from build123d import *

# Parameters (mm, degrees)
SKETCH1_W           = 12.7
SKETCH1_H           = 9.525
BOSS_EXTRUDE1_DEPTH = 2.54
FILLET1_R           = 0.635
SHELL1_START        = 0.635
SHELL1_OUTLINE_W    = 1.905
SHELL1_OUTLINE_H    = 8.255
SHELL1_DEPTH        = 11.43
SKETCH2_R           = 2.54
BOSS_EXTRUDE2_DEPTH = 1.905
BOSS_EXTRUDE3_DEPTH = 0.00254


# Read off the part's stored shape, not the designer's step: Shell1
with BuildPart() as part:
    # Sketch1 → Boss-Extrude1 (new body)
    with BuildSketch(Plane(origin=(0, 0, 0), x_dir=(1, 0, 0), z_dir=(0, 1, 0))):
        with Locations((6.35, 4.7625)):
            Rectangle(SKETCH1_W, SKETCH1_H)
    extrude(amount=BOSS_EXTRUDE1_DEPTH)

    # Fillet1
    fillet1_edges = [part.edges().sort_by_distance(p)[0] for p in [
        (0, 1.27, -9.525),
        (12.7, 1.27, -9.525),
        (12.7, 1.27, 0),
        (0, 1.27, 0),
    ]]
    fillet(fillet1_edges, radius=FILLET1_R)

    # Shell1 outline → Shell1 (cut)
    with BuildSketch(Plane.YZ.offset(SHELL1_START)):
        with Locations((0.9525, -4.7625)):
            Rectangle(SHELL1_OUTLINE_W, SHELL1_OUTLINE_H)
    extrude(amount=SHELL1_DEPTH, mode=Mode.SUBTRACT)

    # Sketch2 → Boss-Extrude2 (add)
    with BuildSketch(Plane(origin=(0, 1.905, 0), x_dir=(-1, 0, 0), z_dir=(0, -1, 0))):
        with Locations(Location((-6.35, 4.7625, 0), (0, 0, 270))):
            Circle(SKETCH2_R)
    extrude(amount=BOSS_EXTRUDE2_DEPTH)

    # Sketch3 → Boss-Extrude3 (add)
    # profile 1 of 3: a face of its own
    with BuildSketch(Plane(origin=(0, 2.54, 0), x_dir=(1, 0, 0), z_dir=(0, 1, 0))):
        Polygon((3.414346154, 6.477), (4.961141026, 6.477), (4.961141026, 5.907128205), (3.984217949, 5.907128205), (3.984217949, 5.296551282), (4.961141026, 5.296551282), (4.961141026, 4.726679487), (3.984217949, 4.726679487), (3.984217949, 3.302), (3.414346154, 3.302), align=None)
    # profile 2 of 3: a face of its own
    with BuildSketch(Plane(origin=(0, 2.54, 0), x_dir=(1, 0, 0), z_dir=(0, 1, 0))):
        Polygon((5.871282252, 6.477), (6.752166667, 6.477), (6.752166667, 3.302), (6.182294872, 3.302), (6.182294872, 5.947833333), (5.531012821, 5.947833333), align=None)
    # profile 3 of 3: a face of its own
    with BuildSketch(Plane(origin=(0, 2.54, 0), x_dir=(1, 0, 0), z_dir=(0, 1, 0))):
        with BuildLine():
            add(Edge.make_bspline(
                [(8.798235377, 6.558410256), (8.825819537, 6.558000762), (8.880057365, 6.557195586), (8.959939478, 6.548474876), (9.036888038, 6.535300314), (9.111204078, 6.516926396), (9.182352664, 6.492609168), (9.25085163, 6.463501864), (9.31588564, 6.428077745), (9.378284086, 6.388064384), (9.438022931, 6.342763586), (9.493666394, 6.291118337), (9.546230643, 6.234316997), (9.594577855, 6.171500832), (9.639778695, 6.10324122), (9.68168464, 6.029527338), (9.719974889, 5.949998406), (9.755078585, 5.864510908), (9.786468421, 5.771783423), (9.812908041, 5.670752326), (9.83558444, 5.561394546), (9.85472492, 5.443437874), (9.869192029, 5.316725518), (9.878943152, 5.181341659), (9.885634834, 5.037547297), (9.886180963, 4.938905546), (9.886461538, 4.888227965)],
                knots=[0, 0, 0, 0, 0.879237366, 1.728815576, 2.559023295, 3.367336655, 4.166867292, 4.954216142, 5.737608147, 6.525189134, 7.316157332, 8.124696809, 8.942788509, 9.781158001, 10.649253743, 11.551476218, 12.482711956, 13.461909668, 14.496590415, 15.601789533, 16.789733467, 18.056700938, 19.410929216, 20.8549011, 22.384193279, 24, 24, 24, 24], degree=3))
            add(Edge.make_bspline(
                [(9.886461538, 4.888227965), (9.886158312, 4.83691635), (9.885569149, 4.737218804), (9.879221327, 4.592109226), (9.86829008, 4.455742398), (9.854201098, 4.32813243), (9.834903048, 4.20934671), (9.812302348, 4.099077662), (9.785445387, 3.997365257), (9.75302158, 3.904438674), (9.718130367, 3.818801041), (9.679735377, 3.739427172), (9.63850583, 3.666102077), (9.595387407, 3.59771955), (9.548016197, 3.53629547), (9.498697891, 3.4797411), (9.445285081, 3.430210667), (9.390026654, 3.385151595), (9.330898269, 3.346211514), (9.268509703, 3.312155161), (9.201748675, 3.284531414), (9.131832125, 3.260505754), (9.057568312, 3.243257923), (8.980137277, 3.229572336), (8.89866484, 3.222008841), (8.843195123, 3.221070539), (8.814771835, 3.220589744)],
                knots=[0, 0, 0, 0, 1.643780988, 3.193836972, 4.651895693, 6.025988579, 7.305620092, 8.505800249, 9.631074763, 10.672816429, 11.65661981, 12.592235626, 13.49536222, 14.350718032, 15.179365177, 15.97804903, 16.751647189, 17.51006938, 18.259804725, 19.016521909, 19.783502495, 20.571750527, 21.382245291, 22.22305063, 23.089471752, 24, 24, 24, 24], degree=3))
            add(Edge.make_bspline(
                [(8.814771835, 3.220589744), (8.786349314, 3.221079814), (8.730670013, 3.222039854), (8.648977266, 3.229516098), (8.571135886, 3.243313364), (8.496284527, 3.26063817), (8.424944142, 3.284478255), (8.356772657, 3.312928485), (8.292294252, 3.346772343), (8.231330396, 3.38580315), (8.174089237, 3.430560743), (8.119681247, 3.480566389), (8.068226781, 3.535693336), (8.020508587, 3.596559051), (7.975745182, 3.662351105), (7.934403375, 3.733820811), (7.896508012, 3.810864109), (7.86087372, 3.893588392), (7.82991203, 3.983774617), (7.802357564, 4.082228137), (7.779785671, 4.189769642), (7.761631843, 4.306364584), (7.747137838, 4.431765951), (7.736355964, 4.566034271), (7.729972884, 4.709232083), (7.729389899, 4.807659072), (7.729089744, 4.858335136)],
                knots=[0, 0, 0, 0, 0.917216111, 1.796812873, 2.643793957, 3.46689424, 4.273913431, 5.068098542, 5.848489301, 6.620921603, 7.401012384, 8.190319798, 9.003608147, 9.831726257, 10.68377682, 11.569763213, 12.493818149, 13.453288342, 14.474581811, 15.568529029, 16.750744269, 18.018426408, 19.375425659, 20.823733699, 22.36466933, 24, 24, 24, 24], degree=3))
            add(Edge.make_bspline(
                [(7.729089744, 4.858335136), (7.729633447, 4.928745538), (7.730682529, 5.064603314), (7.74397727, 5.2608783), (7.763490579, 5.442300526), (7.792151006, 5.608566515), (7.827589229, 5.760292069), (7.872969718, 5.896477699), (7.924632103, 6.019007839), (7.968655093, 6.091595432), (7.989856971, 6.126554287)],
                knots=[0, 0, 0, 0, 1.288568992, 2.486310467, 3.599230591, 4.627010532, 5.572937695, 6.447898582, 7.252493626, 8, 8, 8, 8], degree=3))
            add(Edge.make_bspline(
                [(7.989856971, 6.126554287), (8.014509505, 6.160897855), (8.062710067, 6.228046298), (8.146990098, 6.316199652), (8.237538017, 6.391592717), (8.336213628, 6.452519281), (8.441456335, 6.500565973), (8.5541697, 6.534500812), (8.673937491, 6.554272829), (8.756184031, 6.557010519), (8.798235377, 6.558410256)],
                knots=[0, 0, 0, 0, 1.058512271, 2.069600068, 3.047294572, 4.004278952, 4.967380941, 5.939006123, 6.946246673, 8, 8, 8, 8], degree=3))
        make_face()
        with BuildLine():
            add(Edge.make_bspline(
                [(8.812227764, 5.988538462), (8.787291455, 5.98735653), (8.738403051, 5.985039317), (8.667463648, 5.965369447), (8.600572221, 5.934988272), (8.549689698, 5.898429277), (8.511604636, 5.863383097), (8.48499433, 5.831667444), (8.459332884, 5.796275061), (8.436667403, 5.755608871), (8.415265272, 5.711130059), (8.394348939, 5.662636719), (8.377203038, 5.608937747), (8.360357645, 5.550947646), (8.345599509, 5.487063142), (8.333235426, 5.41676205), (8.322189206, 5.339587196), (8.314484335, 5.25548803), (8.307301083, 5.164552541), (8.302151788, 5.06657816), (8.299998997, 4.961591317), (8.29931469, 4.889288437), (8.298961538, 4.85197496)],
                knots=[0, 0, 0, 0, 1.076674018, 2.110852608, 3.161083442, 4.239746716, 4.804137807, 5.395870207, 6.026861976, 6.692161227, 7.405688833, 8.16177676, 8.973626916, 9.841385931, 10.773283133, 11.807421078, 12.927755683, 14.143907515, 15.458935494, 16.872852025, 18.386167141, 20, 20, 20, 20], degree=3))
            add(Edge.make_bspline(
                [(8.298961538, 4.85197496), (8.299542783, 4.803633547), (8.300657362, 4.710935302), (8.306495007, 4.577631999), (8.318196082, 4.45631526), (8.332749856, 4.346162875), (8.353191227, 4.247889213), (8.376710347, 4.160564514), (8.405754369, 4.085301955), (8.439320333, 4.02101307), (8.476496151, 3.96632265), (8.516852136, 3.919835547), (8.559014312, 3.879579908), (8.604298698, 3.846880749), (8.652597258, 3.821821621), (8.70350679, 3.803796899), (8.757059643, 3.792763217), (8.793732086, 3.7912332), (8.812227764, 3.790461538)],
                knots=[0, 0, 0, 0, 1.771748488, 3.397459088, 4.888034009, 6.237357457, 7.467047327, 8.564189669, 9.548206622, 10.417051504, 11.216568818, 11.965764335, 12.669334354, 13.348544111, 14.005342236, 14.656555988, 15.322436492, 16, 16, 16, 16], degree=3))
            add(Edge.make_bspline(
                [(8.812227764, 3.790461538), (8.83008873, 3.790989566), (8.86505828, 3.79202338), (8.916051715, 3.802635332), (8.96427473, 3.819888063), (9.009581726, 3.844293261), (9.052134759, 3.875328205), (9.091725856, 3.913129275), (9.128056429, 3.95807326), (9.149222786, 3.991428344), (9.160129407, 4.008615585)],
                knots=[0, 0, 0, 0, 0.992283464, 1.942767638, 2.88273346, 3.832339453, 4.79467288, 5.803907806, 6.868395428, 8, 8, 8, 8], degree=3))
            add(Edge.make_bspline(
                [(9.160129407, 4.008615585), (9.172970117, 4.0321014), (9.199896044, 4.08134925), (9.231054773, 4.164453161), (9.257282455, 4.258180636), (9.279856237, 4.362823366), (9.295295327, 4.478794074), (9.308591452, 4.60535738), (9.315004504, 4.743150605), (9.316047621, 4.838614248), (9.316589744, 4.888227965)],
                knots=[0, 0, 0, 0, 0.710965849, 1.490837728, 2.352621235, 3.297892224, 4.334225155, 5.461620853, 6.680770821, 8, 8, 8, 8], degree=3))
            add(Edge.make_bspline(
                [(9.316589744, 4.888227965), (9.316380334, 4.938272352), (9.315977255, 5.034599256), (9.30858193, 5.172887857), (9.298283374, 5.299191543), (9.283219561, 5.41322833), (9.263837227, 5.515275048), (9.239948427, 5.605325026), (9.211785309, 5.683555737), (9.178387208, 5.749889172), (9.141396735, 5.806263493), (9.10213022, 5.854628288), (9.060421626, 5.895920929), (9.016340704, 5.930296808), (8.968867186, 5.956562559), (8.918907879, 5.975108351), (8.866360361, 5.986327934), (8.830515514, 5.987791673), (8.812227764, 5.988538462)],
                knots=[0, 0, 0, 0, 1.793836731, 3.452829483, 4.963243077, 6.335886805, 7.574563692, 8.684454726, 9.672768357, 10.54971625, 11.340229787, 12.085688095, 12.778991901, 13.440269426, 14.083255152, 14.715733572, 15.344777694, 16, 16, 16, 16], degree=3))
        make_face(mode=Mode.SUBTRACT)
    extrude(amount=BOSS_EXTRUDE3_DEPTH)


solid = part.part
Can you work these out from the model? Positions are in its coordinate system, mm. A direction names the side the tool comes from. Coordinates: 2 decimals unless noted, no trailing zeros. Loops run counter-clockwise (first coordinate to the right, second up) from the corner with the lowest first, then second, coordinate; pieces in that order, holes last. Notation, with made-up numbers: M -35,25.25 L -5,25.25 A24 cw -5,39.25 Z; hole C 8,-5 d6. An arc over 180 degrees is marked long. Answer as CSV lines item,"result". Start each with the question number.
1. Suppose I cut it at C-C, the plane z = -1.25. List the corners of the cut face in (x, y) for me (3 decimals).
2. If I drill on probe 1 along Z at (x, y) = (3.5, 0.8) (3 decimals); probe 2 along X at (y, z) = (0.45, -6.75) (3 decimals); probe 3 along Z at (x, y) = (6, 0.1) (3 decimals), over which ranges is the centre line in solid material (lowest first)? Write a range as [from, to].
3. Suppose I cut it at B-B, the plane x = 11.5. List the corners of the cut face in (y, z) for me (3 decimals), plus the area to 3 significant figures.
4. Thinking about a two-plate mould opening in Z: for faces 3 (the face through (6, 1, -9.525)), 4 (the face through (12.7, 1, -5)), 5 (the face through (6, 1, -8.89)), which applies, +Z half, -Z half, draft (parallel to the pull), parting line (faces both ways), or undercut?
5. For faces 1 (the face through (0.635, 1, -5)), 2 (the face through (9.5, 2.543, -4.9)), which set-ups out of +Z, -Z, +X, -X, +Y, -Y let a thin tool reach every point of the face, with its end or its side?
6. Suppose I cut it at A-A, the plane y = 1.1. Count the separate pieces of the cut face and the enclosed holes in it, plus the area to 3 significant figures.
Output:
1,outline,"M 0,0 L 0.635,0 L 0.635,1.905 L 12.065,1.905 L 12.065,0 L 12.7,0 L 12.7,2.54 L 0,2.54 Z"
2,probe 1,"z = [-9.525, -8.89], [-0.635, 0]"
2,probe 2,"x = [0, 0.635], [4.768, 7.932], [12.065, 12.7]"
2,probe 3,"z = [-9.525, -8.89], [-7.278, -2.247], [-0.635, 0]"
3,outline,"M 0,-9.525 L 2.54,-9.525 L 2.54,0 L 0,0 L 0,-0.635 L 1.905,-0.635 L 1.905,-8.89 L 0,-8.89 Z"
3,area,"8.47 mm^2"
4,face 3,"-Z half"
4,face 4,"draft"
4,face 5,"undercut"
5,face 1,"-Y"
5,face 2,"+Z, -Z, +X, -X, +Y"
6,separate pieces,"2"
6,enclosed holes,"1"
6,area,"46.5 mm^2"
